Geometry check sheet. Reference: the model listing, model coordinates, mm. A direction names the side the tool comes from. Round coordinates to 2 decimals unless told otherwise and drop trailing zeros. Write each loop counter-clockwise with the first axis right and the second up, starting at its lowest first coordinate (ties: lowest second). Pieces come first, ordered by that corner, then holes.
Autodesk Inventor part; units mm, degrees
ref_plane "YZ Plane" through (0, 0, 0) normal (1, 0, 0) x (0, 1, 0)
ref_plane "XZ Plane" through (0, 0, 0) normal (0, 1, 0) x (-1, 0, 0)
ref_plane "XY Plane" through (0, 0, 0) normal (0, 0, 1) x (1, 0, 0)
sketch "Esboço1" plane through (0, 0, 0) normal (0, 1, 0) x (-1, 0, 0)
  line L0 (0, 0) -> (-113, 0)
  line L1 (-113, 0) -> (-113, -34)
  line L2 (-113, -34) -> (0, -34)
  line L3 (0, -34) -> (0, 0)
  line L4 (0, 0) -> (-7, 0)
  line L5 (0, -11) -> (0, 0)
  circle A0 centre (-7, -11) radius 2.25
  circle A1 centre (-7, -23) radius 2.25
  circle A2 centre (-31, -11) radius 2.25
  circle A3 centre (-31, -23) radius 2.25
  line L6 (-56.5, 0) -> (-56.5, -13.25)
  circle A4 centre (-106, -11) radius 2.25
  circle A5 centre (-106, -23) radius 2.25
  circle A6 centre (-82, -23) radius 2.25
  circle A7 centre (-82, -11) radius 2.25
  circle A8 centre (-7, -11) radius 3.5
  circle A9 centre (-7, -23) radius 3.5
  circle A10 centre (-31, -23) radius 3.5
  circle A11 centre (-31, -11) radius 3.5
  circle A12 centre (-106, -11) radius 3.5
  circle A13 centre (-106, -23) radius 3.5
  circle A14 centre (-82, -23) radius 3.5
  circle A15 centre (-82, -11) radius 3.5
  dimension "d0" = 113
  dimension "d1" = 34
  dimension "d6" = 7
  dimension "d7" = 7
  dimension "d8" = 7
  dimension "d9" = 7
extrude "Extrusão1" add sketch "Esboço1" along normal blind 1 contours L3 L2 L1 L0
sketch "Esboço2" plane through (0, 1, 0) normal (0, 1, 0) x (1, 0, 0)
  circle A0 centre (7, 11) radius 3.5
  circle A1 centre (7, 11) radius 3.5
  circle A2 centre (7, 23) radius 3.5
  circle A3 centre (7, 23) radius 3.5
  circle A4 centre (31, 23) radius 3.5
  circle A5 centre (31, 23) radius 3.5
  circle A6 centre (31, 11) radius 3.5
  circle A7 centre (31, 11) radius 3.5
  circle A8 centre (82, 23) radius 3.5
  circle A9 centre (82, 23) radius 3.5
  circle A10 centre (106, 23) radius 3.5
  circle A11 centre (106, 23) radius 3.5
  circle A12 centre (106, 11) radius 3.5
  circle A13 centre (106, 11) radius 3.5
  circle A14 centre (82, 11) radius 3.5
  circle A15 centre (82, 11) radius 3.5
  point P0 (0, 0)
extrude "Extrusão2" add sketch "Esboço2" against normal blind 2 contours A0 | A2 | A4 | A6 | A8 | A14
sketch "Esboço3" plane through (0, 1, 0) normal (0, 1, 0) x (1, 0, 0)
  circle A0 centre (106, 11) radius 3.5
  circle A1 centre (106, 11) radius 3.5
  circle A2 centre (106, 23) radius 3.5
  circle A3 centre (106, 23) radius 3.5
  point P0 (0, 0)
extrude "Extrusão3" add sketch "Esboço3" against normal blind 2
sketch "Esboço4" plane through (7, -1, -11) normal (0, -1, 0) x (1, 0, 0)
  circle A0 centre (0, 0) radius 3.5
  circle A1 centre (0, 0) radius 2.25
  line L0 (106, -23) -> (-7, -23)
  line L1 (49.5, -23) -> (49.5, -11.349)
  line L2 (0, -23) -> (12, -23)
  line L3 (12, -23) -> (12, -13.2533)
  line L4 (-7, -23) -> (-7, 11)
  line L5 (-7, -6) -> (6, -6)
  circle A2 centre (0, -12) radius 2.25
  circle A3 centre (24, 0) radius 2.25
  circle A4 centre (24, -12) radius 2.25
  circle A5 centre (99, 0) radius 2.25
  circle A6 centre (99, -12) radius 2.25
  circle A7 centre (75, 0) radius 2.25
  circle A8 centre (75, -12) radius 2.25
  dimension "d16" = 4.5
  dimension "d17" = 12
extrude "Extrusão4" add sketch "Esboço4" along normal blind 2.5 contours A1 | A2 | A3 | A4 | A5 | A6 | A7 | A8
sketch "Esboço5" plane through (7, -3.5, -11) normal (0, -1, 0) x (1, 0, 0)
  line L0 (0.0116, -1.5787) -> (-1.3614, -0.7993)
  line L1 (-1.3614, -0.7993) -> (-1.373, 0.7793)
  line L2 (-1.373, 0.7793) -> (-0.0116, 1.5787)
  line L3 (-0.0116, 1.5787) -> (1.3614, 0.7993)
  line L4 (1.3614, 0.7993) -> (1.373, -0.7793)
  line L5 (1.373, -0.7793) -> (0.0116, -1.5787)
  line L6 (-7, -23) -> (-7, 11)
  circle A0 centre (0, -12) radius 3.5
  line L7 (106, -23) -> (-7, -23)
  line L8 (0.0116, -10.4213) -> (-1.3614, -11.2007)
  line L9 (-1.3614, -11.2007) -> (-1.373, -12.7793)
  line L10 (-1.373, -12.7793) -> (-0.0116, -13.5787)
  line L11 (-0.0116, -13.5787) -> (1.3614, -12.7993)
  line L12 (1.3614, -12.7993) -> (1.373, -11.2207)
  line L13 (1.373, -11.2207) -> (0.0116, -10.4213)
  line L14 (23.9884, -1.5787) -> (25.3614, -0.7993)
  line L15 (25.3614, -0.7993) -> (25.373, 0.7793)
  line L16 (25.373, 0.7793) -> (24.0116, 1.5787)
  line L17 (24.0116, 1.5787) -> (22.6386, 0.7993)
  line L18 (22.6386, 0.7993) -> (22.627, -0.7793)
  line L19 (22.627, -0.7793) -> (23.9884, -1.5787)
  line L20 (23.9884, -10.4213) -> (25.3614, -11.2007)
  line L21 (25.3614, -11.2007) -> (25.373, -12.7793)
  line L22 (25.373, -12.7793) -> (24.0116, -13.5787)
  line L23 (22.6386, -12.7993) -> (22.627, -11.2207)
  line L24 (22.627, -11.2207) -> (23.9884, -10.4213)
  line L25 (24.0116, -13.5787) -> (22.6386, -12.7993)
  line L26 (98.9884, -1.5787) -> (100.3614, -0.7993)
  line L27 (100.3614, -0.7993) -> (100.373, 0.7793)
  line L28 (100.373, 0.7793) -> (99.0116, 1.5787)
  line L29 (99.0116, 1.5787) -> (97.6386, 0.7993)
  line L30 (97.6386, 0.7993) -> (97.627, -0.7793)
  line L31 (97.627, -0.7793) -> (98.9884, -1.5787)
  line L32 (98.9884, -10.4213) -> (100.3614, -11.2007)
  line L33 (100.3614, -11.2007) -> (100.373, -12.7793)
  line L34 (100.373, -12.7793) -> (99.0116, -13.5787)
  line L35 (97.6386, -12.7993) -> (97.627, -11.2207)
  line L36 (97.627, -11.2207) -> (98.9884, -10.4213)
  line L37 (99.0116, -13.5787) -> (97.6386, -12.7993)
  line L38 (75.0116, -10.4213) -> (73.6386, -11.2007)
  line L39 (76.373, -11.2207) -> (75.0116, -10.4213)
  line L40 (73.6386, -11.2007) -> (73.627, -12.7793)
  line L41 (76.3614, -12.7993) -> (76.373, -11.2207)
  line L42 (74.9884, -13.5787) -> (76.3614, -12.7993)
  line L43 (73.627, -12.7793) -> (74.9884, -13.5787)
  line L44 (76.373, -0.7793) -> (75.0116, -1.5787)
  line L45 (73.6386, -0.7993) -> (73.627, 0.7793)
  line L46 (76.3614, 0.7993) -> (76.373, -0.7793)
  line L47 (73.627, 0.7793) -> (74.9884, 1.5787)
  line L48 (74.9884, 1.5787) -> (76.3614, 0.7993)
  line L49 (75.0116, -1.5787) -> (73.6386, -0.7993)
  point P0 (0, 0)
  point P1 (24, 0)
  point P2 (24, -12)
  point P3 (99, 0)
  point P4 (75, 0)
  point P5 (75, -12)
extrude "Extrusão5" cut sketch "Esboço5" against normal blind 1.5 contours L0 L1 L2 L3 L4 L5 | L13 L12 L11 L10 L9 L8 | L19 L18 L17 L16 L15 L14 | L20 L21 L22 L25 L23 L24 | L31 L30 L29 L28 L27 L26 | L32 L33 L34 L37 L35 L36 | L39 L41 L42 L43 L40 L38 | L44 L49 L45 L47 L48 L46
sketch "Esboço6" plane through (0, 0, 0) normal (0, -1, 0) x (1, 0, 0)
  point P0 (0, 0)
properties part number "chapinha_garra"
1. Scan lines: line 1 along X through (y, z) = (-1.25, -21.5); line 2 along X through (y, z) = (-0.7, -20.5); line 3 along Y through (x, z) = (47.5, -4). Record each from-to range of solid material in increasing order.
2. Depth check by flat-ended pin: pin 1 Ø2 at (x, z) = (7, -23) entering from -Y; pin 2 Ø5.5 at (x, z) = (7, -23) entering from -Y; pin 3 Ø17 at (x, z) = (54.5, -24) entering from -Y. Enter the tip coordinate at first touch or a pass-through.
3. Section check A-A (x = 47). Record the cut outline in (y, z).
4. Access from +Z, -Z, +X, -X, +Y, -Y to the whole of each face (thin tool, end or side, straight path). Record for faces 1 (the face through (7.5, -3.5, -12.5)), 2 (the face through (108.3, -1, -10.3)).
5. Section check B-B (z = -2.5). Record the cut outline in (x, y).
6. Release check for a two-part mould opening along Z. For faces 3 (the face through (82.5, -3.5, -12.5)), 4 (the face through (31.7, -1, -8.7)) record: +Z half, -Z half, draft (parallel to the pull), parting line (faces both ways), or undercut.
Results below:
1. line 1: x = 5.32 to 8.68, 29.32 to 32.68, 80.32 to 83.68, 104.32 to 107.68
1. line 2: x = 4.55 to 9.45, 28.55 to 33.45, 79.55 to 84.45, 103.55 to 108.45
1. line 3: y = 0 to 1
2. pin 1: stops at y = -2
2. pin 2: stops at y = -3.5
2. pin 3: stops at y = 0
3. outline: (0, -34) - (1, -34) - (1, 0) - (0, 0) - close
4. face 1: +Z, -Z, +X, -X, -Y
4. face 2: -Y
5. outline: (0, 0) - (113, 0) - (113, 1) - (0, 1) - close
6. face 3: draft
6. face 4: undercut
